```python
from build123d import *

# Parameters (mm, degrees)
BOSS_EXTRUDE1_DEPTH = 3.175
SKETCH2_R           = 12.7
CUT_EXTRUDE1_DEPTH  = 64.579325453
FILLET1_R           = 2.54


with BuildPart() as part:
    # Sketch1 → Boss-Extrude1 (new body)
    with BuildSketch(Plane(origin=(0, 0, 0), x_dir=(1, 0, 0), z_dir=(0, 1, 0))):
        with BuildLine():
            Line((-9.498044736, 8.430726315), (-50.8, -38.1))
            Line((-50.8, -38.1), (-16.8372204, -38.1))
            Line((-16.8372204, -38.1), (9.498044736, -8.430726315))
            ThreePointArc((9.498044736, -8.430726315), (8.430726315, 9.498044736), (-9.498044736, 8.430726315))
        make_face()
    extrude(amount=BOSS_EXTRUDE1_DEPTH)

    # Sketch2 → Cut-Extrude1 (cut, through all)
    with BuildSketch(Plane.XZ):
        Circle(SKETCH2_R)
    extrude(amount=-CUT_EXTRUDE1_DEPTH, mode=Mode.SUBTRACT)

    # Fillet1
    fillet1_edges = [part.edges().sort_by_distance(p)[0] for p in [
        (9.498044736, 1.5875, 8.430726315),
    ]]
    fillet(fillet1_edges, radius=FILLET1_R)
    fillet1_2_edges = [part.edges().sort_by_distance(p)[0] for p in [
        (-9.498044736, 1.5875, -8.430726315),
    ]]
    fillet(fillet1_2_edges, radius=FILLET1_R)


solid = part.part
```
The listing builds one solid part. Answer for the finished solid, in the listing's coordinates (mm). Give positions to 0.01 mm unless a question says otherwise; leave off trailing zeros. Order: outer loops, then holes, each group sorted by start corner. A loop starts at its lowest first (then second) coordinate and runs counter-clockwise, first axis right, second up. Notation, with made-up numbers: (55.5, 39) -> (84.5, 39) arc R21 ccw to (84.5, 62) -> close; hole circle Ø6 at (-37, -39). An arc over 180 degrees is marked (long way). Answer as CSV lines item,"result". Start each with the question number.
Q1. Find the intervals of material crossed by L1, parallel to Z at x = -43.5, y = 2.1; L2, parallel to Z at x = -39.5, y = 2.15; L3, parallel to X at y = 0.65, z = 10, in increasing order.
Q2. A cutting plane is placed at B-B (z = 7.5). Determine the outline of the cut face in (x, y) (3 decimals).
Q3. A cutting plane is placed at A-A (x = -21). Determine the outline of the cut face in (y, z) (3 decimals), then the cut area to 3 significant figures.
Q4. Determine the mould class of faces 1 (the cylindrical face through (2.355, 1.61, 14.157)), 2 (the flat face through (-33.683, 1.565, 18.816)), 3 (the flat face through (-24, 0, 23)), 4 (the flat face through (-34, 2, 38.1)) for opening direction Z: pulls with the +Z half, pulls with the -Z half, needs draft (parallel to the pull), parting line crosses it, or undercut.
Results found:
1,L1,"29.88 to 38.1"
1,L2,"25.37 to 38.1"
1,L3,"-25.86 to -7.83"
2,outline,"(-23.639, 0) -> (-10.249, 0) -> (-10.249, 3.175) -> (-23.639, 3.175) -> close"
3,outline,"(0, 4.527) -> (3.175, 4.527) -> (3.175, 38.1) -> (0, 38.1) -> close"
3,area,"107 mm2"
4,face 1,"parting line crosses it"
4,face 2,"pulls with the -Z half"
4,face 3,"needs draft"
4,face 4,"pulls with the +Z half"
